```python
from build123d import *

# Parameters (mm, degrees)
F0_W     = 400
F0_H     = 50
F1_DEPTH = 25
F2_R     = 4
F3_DEPTH = 25
F4_W     = 60
F4_H     = 35
F5_DEPTH = 5
F6_R     = 2.5
F7_DEPTH = 30.001
F8_R     = 1.5


with BuildPart() as f1:
    # F0 (on Front) → F1 (new body)
    with BuildSketch(Plane.XZ):
        Rectangle(F0_W, F0_H)
    extrude(amount=F1_DEPTH)

    # F2 (on face) → F3 (cut, through all)
    with BuildSketch(Plane.XZ.offset(25)):
        with Locations((-187.5, 10)):
            Circle(F2_R)
        with Locations((-187.5, -10)):
            Circle(F2_R)
        with Locations((187.5, 10)):
            Circle(F2_R)
        with Locations((187.5, -10)):
            Circle(F2_R)
    extrude(amount=-F3_DEPTH, mode=Mode.SUBTRACT)

    # F4 (on face) → F5 (join)
    with BuildSketch(Plane(origin=(0, 0, 0), x_dir=(-1, 0, 0), z_dir=(0, 1, 0))):
        Rectangle(F4_W, F4_H)
    extrude(amount=F5_DEPTH)

    # F6 (on face) → F7 (cut, through all)
    with BuildSketch(Plane(origin=(0, 5, 0), x_dir=(-1, 0, 0), z_dir=(0, 1, 0))):
        with Locations((-25, 12.5)):
            Circle(F6_R)
        with Locations((25, 12.5)):
            Circle(F6_R)
        with Locations((25, -12.5)):
            Circle(F6_R)
        with Locations((-25, -12.5)):
            Circle(F6_R)
    extrude(amount=-F7_DEPTH, mode=Mode.SUBTRACT)

    # F11: sweep along a path in F10
    with BuildLine(Plane.XY) as f11_path:
        ThreePointArc((5, 5), (0, 10), (-5, 5))
    # F8 (on face) → F11 (sweep)
    with BuildSketch(Plane(origin=(0, 5, 0), x_dir=(-1, 0, 0), z_dir=(0, 1, 0))):
        with Locations((-5, 0)):
            Circle(F8_R)
    sweep(path=f11_path.line)


solid = f1.part
```
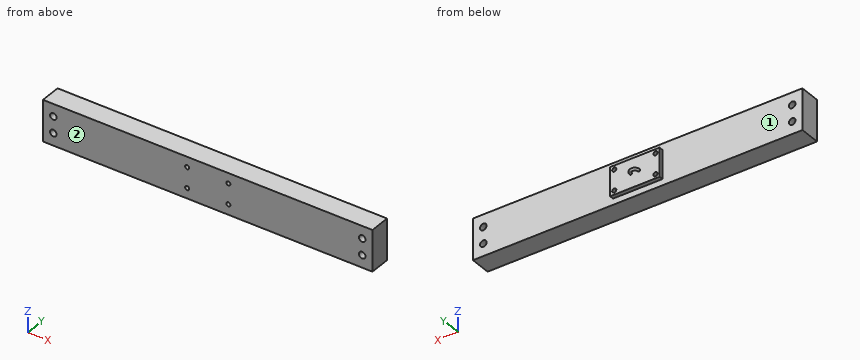
Verification items for the finished model (mm, model axes). Face numbers are marked on the shaded views. Coordinates: 2 decimals unless noted, no trailing zeros. Write each loop counter-clockwise with the first axis right and the second up, starting at its lowest first coordinate (ties: lowest second). Pieces come first, ordered by that corner, then holes. Notation, with made-up numbers: M -29.5,-9 L -17.5,-9 A22 cw -17.5,20 Z; hole C 81.25,43.5 d1. An arc over 180 degrees is marked long. Answer as a JSON object with one key per item and string values. Group by question number.
(1) Release check for a two-part mould opening along Y. For the marked faces 1 and 2 record: +Y half, -Y half, draft (parallel to the pull), parting line (faces both ways), or undercut.
(2) Gauge pin test, flat ends, axial feed: pin 1 (6 mm diameter, centred on x = -25, z = -12.5, fed in from +Y); pin 2 (9 mm diameter, centred on x = -187.5, z = -10, fed in from +Y); pin 3 (1.5 mm diameter, centred on y = 4, z = -15, fed in from +X); pin 4 (4 mm diameter, centred on x = -25, z = 12.5, fed in from +Y). Record the tip position at first contact, or that the pin passes through.
(3) Cross-section at A-A, the plane x = -187.5. Record the cut outline in (y, z), and give its area (3 significant figures).
(4) Material ranges on line 1 (Z direction, x = 25, y = -16); line 2 (Z direction, x = 187.5, y = -5.5); line 3 (X direction, y = -17, z = 12), recorded low to high.
Reply:
{
 "1": {"face 1": "+Y half", "face 2": "-Y half"},
 "2": {"pin 1": "y = 5", "pin 2": "y = 0", "pin 3": "x = 30", "pin 4": "through"},
 "3": {"outline": "M -25,-25 L 0,-25 L 0,-14 L -25,-14 Z; M -25,-6 L 0,-6 L 0,6 L -25,6 Z; M -25,14 L 0,14 L 0,25 L -25,25 Z", "area": "850 mm²"},
 "4": {"line 1": "-25 to -15, -10 to 10, 15 to 25", "line 2": "-25 to -14, -6 to 6, 14 to 25", "line 3": "-200 to -190.96, -184.04 to -27.45, -22.55 to 22.55, 27.45 to 184.04, 190.96 to 200"}
}
